CAD build for the part. Positions are in the model's coordinates, mm. Face numbers are marked on the shaded views. Round coordinates to 2 decimals unless told otherwise and drop trailing zeros. Answer as CSV lines item,"result". Start each with the question number.
from build123d import *

# Parameters (mm, degrees)
EXTRUDE_1_DEPTH          = 4
EXTRUDE_2_DEPTH          = 0.25
PATTERN_CIRCULAR_1_COUNT = 2
SKETCH_4_R               = 0.85
CUT_EXTRUDE_1_DEPTH      = 5.0000001


with BuildPart() as part:
    # 草图1 → 凸台-拉伸1 (new body)
    with BuildSketch(Plane(origin=(0, 0, 0), x_dir=(1, 0, 0), z_dir=(0, 1, 0))):
        with BuildLine():
            ThreePointArc((4.545454545, 1.947662299), (0, 1.424285286), (-4.545454545, 1.947662299))
            ThreePointArc((-4.545454545, 1.947662299), (-7, 0), (-4.545454545, -1.947662299))
            ThreePointArc((-4.545454545, -1.947662299), (0, -1.424285286), (4.545454545, -1.947662299))
            ThreePointArc((4.545454545, -1.947662299), (7, 0), (4.545454545, 1.947662299))
        make_face()
    extrude(amount=EXTRUDE_1_DEPTH)

    # 草图3 → 凸台-拉伸2 (add, symmetric)
    with BuildSketch(Plane(origin=(0, 1.866025404, 0.5), x_dir=(0, 0.258819045, -0.965925826), z_dir=(0, -0.965925826, -0.258819045))):
        with BuildLine():
            Line((-0.721025856, 5), (-3.244156646, 8.963824719))
            ThreePointArc((-3.244156646, 8.963824719), (-3.530742288, 9.544023278), (-3.686238371, 10.172181433))
            add(Edge.make_bspline(
                [(-3.686238371, 10.172181433), (-4.525441011, 16.369200543), (-3.695143097, 32.261586596), (-4.002824546, 48.145456087), (-2.214031519, 58.654900349)],
                knots=[0.01661138, 0.01661138, 0.01661138, 0.01661138, 0.374640407, 0.984355774, 0.984355774, 0.984355774, 0.984355774], degree=3))
            ThreePointArc((-2.214031519, 58.654900349), (-1.881256083, 59.24442325), (-1.249204631, 59.486885007))
            ThreePointArc((-1.249204631, 59.486885007), (-0.196436424, 59.499675736), (0.85639329, 59.493836576))
            ThreePointArc((0.85639329, 59.493836576), (1.46199409, 59.278546742), (1.811474117, 58.739134328))
            add(Edge.make_bspline(
                [(1.931851653, 5), (5.579965015, 23.055167147), (6.356652938, 40.76793724), (1.811474117, 58.739134328)],
                knots=[0, 0, 0, 0, 0.986483201, 0.986483201, 0.986483201, 0.986483201], degree=3))
            Line((1.931851653, 5), (-0.721025856, 5))
        make_face()
    extrude_2 = extrude(amount=EXTRUDE_2_DEPTH, both=True)

    # 阵列(圆周)1: 凸台-拉伸2 ×2 about axis
    pattern_circular_1_axis = Axis((0, 4.2, 0), (0, -1, 0))
    for i in range(1, PATTERN_CIRCULAR_1_COUNT):
        add(extrude_2.rotate(pattern_circular_1_axis, i * 360 / PATTERN_CIRCULAR_1_COUNT))

    # 草图4 → 切除-拉伸1 (cut, through all)
    with BuildSketch(Plane(origin=(0, 4, 0), x_dir=(1, 0, 0), z_dir=(0, 1, 0))):
        with Locations((-5, 0)):
            Circle(SKETCH_4_R)
        with Locations((5, 0)):
            Circle(SKETCH_4_R)
    extrude(amount=-CUT_EXTRUDE_1_DEPTH, mode=Mode.SUBTRACT)


solid = part.part
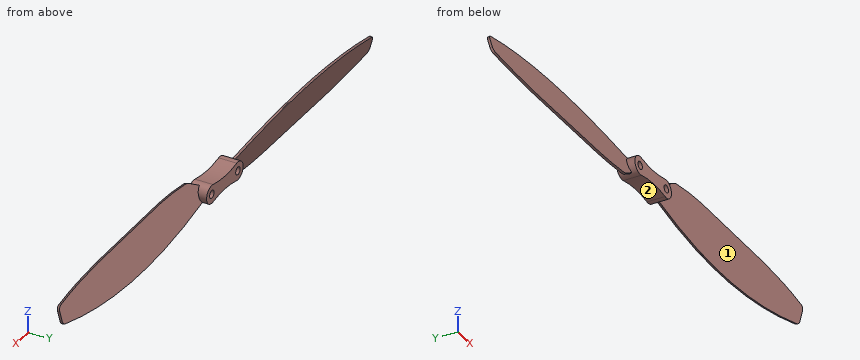
Item 1: Mould opens along X. For the marked faces 1 and 2 say: released by +X, released by -X, zero draft, split by the parting line, or undercut.
Item 2: Probe line 1 (X direction, y = 2.1, z = 0); line 2 (X direction, y = 3.15, z = 0); line 3 (Z direction, x = 5, y = 2.45). List the from-to ranges inside material, lowest first.
Item 3: Pin check, flat tips, straight feed: pin 1 (1 mm diameter, centred on x = -5, y = 0.5, fed in from +Z); pin 2 (2 mm diameter, centred on x = -13.5, z = 3.5, fed in from -Y). Stop position of each tip, or through.
Values:
1,face 1,"zero draft"
1,face 2,"undercut"
2,line 1,"-59.5 to -5.85, -4.15 to 4.15, 5.85 to 59.5"
2,line 2,"-7 to -5.85, -4.15 to 4.15, 5.85 to 7"
2,line 3,"-2 to -0.85, 0.85 to 2"
3,pin 1,"z = 2"
3,pin 2,"y = 2.41"
